Part model, mm, in its own coordinate system. Face numbers are marked on the shaded views. A direction names the side the tool comes from. Round coordinates to 2 decimals unless told otherwise and drop trailing zeros. Write each loop counter-clockwise with the first axis right and the second up, starting at its lowest first coordinate (ties: lowest second). Pieces come first, ordered by that corner, then holes. Notation, with made-up numbers: M -30.5,86 L -18.5,86 A26 ccw -18.5,108 Z; hole C 24.5,72 d11. An arc over 180 degrees is marked long. Answer as a JSON object with one key per item and string values. Group by question number.
1. Band-saw the part on A-A, the plane z = 0. Write the cut outline in (x, y), plus the area to 4 significant figures.
2. Drop flat-ended pins along their axis: pin 1 (2 mm diameter, centred on y = -7.5, z = 3.5, fed in from +X); pin 2 (5 mm diameter, centred on y = 2.5, z = 12, fed in from +X); pin 3 (8 mm diameter, centred on x = -3, y = 10, fed in from -Z); pin 4 (6 mm diameter, centred on x = -6, y = 6.5, fed in from +Z). Give the stop position or say it passes through.
3. Two-plate mould, pull along Y, no slides. Class the marked faces 1, 2 and 3: +Y half, -Y half, draft (parallel to the pull), parting line (faces both ways), or undercut.
4. Drill centre lines: line 1 (Y direction, x = 4.5, z = 9.5); line 2 (X direction, y = -6, z = 3.75); line 3 (Y direction, x = 6, z = -1.5). Where is each one in solid material? Low to high. Write a range as from..to.
5. Band-saw the part on D-D, the plane z = -5.75. Write the cut outline in (x, y).
6. Band-saw the part on C-C, the plane x = -4.5. Write the cut outline in (y, z), plus the area to 3 significant figures.
7. Which spindle directions (+Z, -Z, +X, -X, +Y, -Y) get a long thin tool onto all of the face, cutting with end or side? Do the marked faces 4, 5 and 6. Say none if no direction does.
Autodesk Inventor part; units mm, degrees
ref_plane "YZ Plane" through (0, 0, 0) normal (1, 0, 0) x (0, 1, 0)
ref_plane "XZ Plane" through (0, 0, 0) normal (0, 1, 0) x (-1, 0, 0)
ref_plane "XY Plane" through (0, 0, 0) normal (0, 0, 1) x (1, 0, 0)
sketch "Esboço1" plane through (0, 0, 0) normal (1, 0, 0) x (0, 1, 0)
  circle A0 centre (0, 0) radius 15
  dimension "d0" = 30
extrude "Extrusão1" add sketch "Esboço1" along normal mid plane 15
sketch "Esboço2" plane through (7.5, 0, 0) normal (1, 0, 0) x (0, 0, -1)
  circle A0 centre (0, 0) radius 12.5
  dimension "d3" = 25
extrude "Extrusão2" cut sketch "Esboço2" along normal through all both and the other way through all
ref_plane "Plano de trabalho1" through (0, 0, 0) normal (1, 0, 0) x (0, 0, -1)
sketch "Esboço3" plane through (0, 0, 0) normal (1, 0, 0) x (0, 0, -1)
  circle A0 centre (0, 0) radius 13.75
  dimension "d6" = 27.5
extrude "Extrusão3" add sketch "Esboço3" along normal mid plane 7.5
sketch "Esboço4" plane through (-3.75, 0, 0) normal (-1, 0, 0) x (0, 0, 1)
  circle A0 centre (0, 0) radius 2.5
  dimension "d9" = 5
extrude "Extrusão4" cut sketch "Esboço4" against normal blind 3
properties part number "RodaG" material "Borracha"
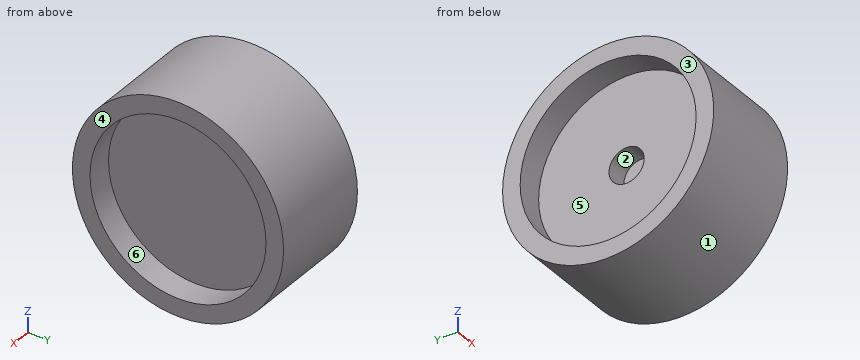
Worked answers:
{
 "1": {"outline": "M -7.5,-15 L 7.5,-15 L 7.5,-12.5 L 3.75,-12.5 L 3.75,12.5 L 7.5,12.5 L 7.5,15 L -7.5,15 L -7.5,12.5 L -3.75,12.5 L -3.75,2.5 L -0.75,2.5 L -0.75,-2.5 L -3.75,-2.5 L -3.75,-12.5 L -7.5,-12.5 Z", "area": "247.5 mm^2"},
 "2": {"pin 1": "stops at x = 3.75", "pin 2": "stops at x = 7.5", "pin 3": "stops at z = -13.75", "pin 4": "stops at z = 14.59"},
 "3": {"face 1": "parting line", "face 2": "undercut", "face 3": "draft"},
 "4": {"line 1": "y = -11.61..-8.12, 8.12..11.61", "line 2": "x = -3.75..3.75", "line 3": "y = -14.92..-12.41, 12.41..14.92"},
 "5": {"outline": "M -7.5,-13.85 L 7.5,-13.85 L 7.5,-11.1 L 3.75,-11.1 L 3.75,11.1 L 7.5,11.1 L 7.5,13.85 L -7.5,13.85 L -7.5,11.1 L -3.75,11.1 L -3.75,-11.1 L -7.5,-11.1 Z"},
 "6": {"outline": "C 0,0 d30; hole C 0,0 d25", "area": "216 mm^2"},
 "7": {"face 4": "+Z, -Z, +X, +Y, -Y", "face 5": "-X", "face 6": "+X"}
}
